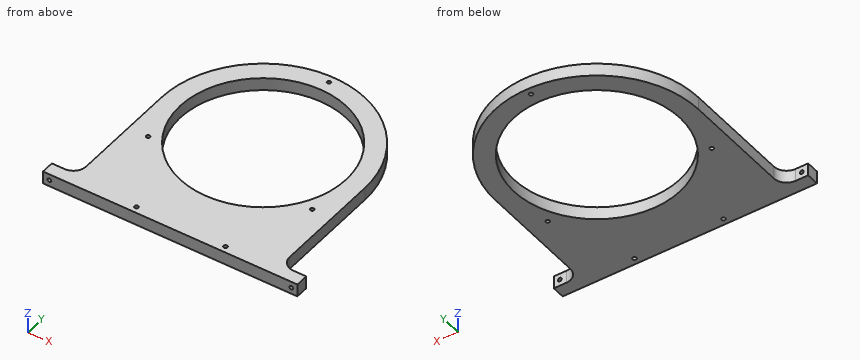
Autodesk Fusion 360 part; units mm, degrees
sketch "Sketch1" plane through (0, 0, 0) normal (0, 0, 1) x (1, 0, 0)
  circle A0 centre (0, 0) radius 65.25
  circle A1 centre (0, 0) radius 74.419 construction
  circle A2 centre (0, 74.419) radius 1.5
  circle A3 centre (-64.4487, -37.2095) radius 1.5
  circle A4 centre (64.4487, -37.2095) radius 1.5
  circle A5 centre (0, 0) radius 80
  line L0 (-80, 0) -> (80, 0) construction
  line L1 (-80, 0) -> (-80, -85)
  line L2 (80, -85) -> (80, 0)
  line L3 (-80, -95) -> (-100, -95) construction
  line L4 (-100, -95) -> (-90, -95)
  line L5 (100, -95) -> (100, -105)
  line L6 (100, -105) -> (-100, -105)
  line L7 (-100, -105) -> (-100, -95)
  arc A6 (-90, -95) -> (-80, -85) centre (-90, -85) ccw
  line L8 (90, -95) -> (100, -95)
  arc A7 (80, -85) -> (90, -95) centre (90, -85) ccw
  line L9 (-100, -100) -> (-30, -100) construction
  line L10 (-100, -100) -> (40, -100) construction
  circle A8 centre (-30, -100) radius 1.5
  circle A9 centre (40, -100) radius 1.5
  dimension "d1" = 130.5
  dimension "d4" = 148.838
  dimension "d5" = 3
  dimension "d7" = 360
  dimension "d8" = 160
  dimension "d10" = 200
  dimension "d11" = 10
  dimension "d12" = 10
  dimension "d13" = 10
  dimension "d22" = 105
  dimension "d24" = 70
  dimension "d25" = 140
  dimension "d26" = 3
  dimension "d27" = 3
extrude "Extrude1" add sketch "Sketch1" along normal blind 10
hole "Hole1" at (-95, -95, 5) direction (0, -1, 0) diameter 3 depth 10 tip angle 118
hole "Hole2" at (95.1862, -95, 5.0204) direction (0, -1, 0) diameter 3 depth 10 tip angle 118
equation "d1 = GearboxDia + Tollerance"
equation "GearboxDia = 130 mm"
equation "Tollerance = 0.5 mm"
equation "d4 = ( 74.419 * 2 ) * 1 mm"
equation "d8 = GearboxDia + 30 mm"
equation "d10 = d8 + 40 mm"
equation "d22 = AxleHieght"
equation "AxleHieght = 105 mm"
equation "d24 = ( 210 / 3 ) * 1 mm"
equation "d25 = ( 210 / 3 * 2 ) * 1 mm"
CAD build for the part. Positions are in the model's coordinates, mm. Give positions to 0.01 mm unless a question says otherwise; leave off trailing zeros. Write each loop counter-clockwise with the first axis right and the second up, starting at its lowest first coordinate (ties: lowest second). Pieces come first, ordered by that corner, then holes. Notation, with made-up numbers: (82.25, 4) - (98.25, 4) arc R18 ccw to (98.25, 26) - close; hole circle Ø6 at (22.25, 52). An arc over 180 degrees is marked (long way). Answer as CSV lines item,"result".
Q1. Band-saw the part on A-A (y = -6). Give the cut face in (x, z), and give its area (3 significant figures).
Result set:
outline,"(-80, 0) - (-64.97, 0) - (-64.97, 10) - (-80, 10) - close; (64.97, 0) - (80, 0) - (80, 10) - (64.97, 10) - close"
area,"301 mm²"
Q2. Flat gauge pins, fed straight in: pin 1 Ø2.5 at (x, y) = (64.45, -37.21) entering from +Z; pin 2 Ø6 at (y, z) = (-53.5, 9) entering from +X; pin 3 Ø1 at (y, z) = (24.5, 9) entering from +X; pin 4 Ø3 at (x, z) = (93, 3.5) entering from +Y. Where does each tip first touch, or does it go through?
Result set:
pin 1,"through"
pin 2,"x = 80"
pin 3,"x = 76.32"
pin 4,"y = -95"
Q3. Band-saw the part on C-C (z = 8.5). Give the cut face in (x, y).
Result set:
outline,"(-100, -105) - (100, -105) - (100, -95) - (90, -95) arc R10 cw to (80, -85) - (80, 0) arc R80 ccw to (-80, 0) - (-80, -85) arc R10 cw to (-90, -95) - (-100, -95) - close; hole circle Ø3 at (-64.45, -37.21); hole circle Ø130.5 at (0, 0); hole circle Ø3 at (-30, -100); hole circle Ø3 at (0, 74.42); hole circle Ø3 at (40, -100); hole circle Ø3 at (64.45, -37.21)"
Q4. Band-saw the part on D-D (y = -91). Give the cut face in (x, z), and give its area (3 significant figures).
Result set:
outline,"(-82, 0) - (82, 0) - (82, 10) - (-82, 10) - close"
area,"1,640 mm²"
Q5. Drill centre lines: line 1 (Y direction, x = 0, z = 5); line 2 (X direction, y = -96.75, z = 5); line 3 (X direction, y = -100, z = 5.5). Where is each one in solid material? Low to high. Write a range as from..to.
Result set:
line 1,"-105..-65.25, 65.25..72.92, 75.92..80"
line 2,"-100..-96.5, -93.5..93.69, 96.69..100"
line 3,"-100..-96.41, -93.59..-31.5, -28.5..38.5, 41.5..93.76, 96.61..100"
Q6. Band-saw the part on B-B (x = -7). Give the cut face in (y, z).
Result set:
outline,"(-105, 0) - (-64.87, 0) - (-64.87, 10) - (-105, 10) - close; (64.87, 0) - (79.69, 0) - (79.69, 10) - (64.87, 10) - close"
